Read the model definition and answer for the solid it produces. Units are mm, in the model's axes. A direction names the side the tool comes from. Coordinates: 2 decimals unless noted, no trailing zeros. Order: outer loops, then holes, each group sorted by start corner. A loop starts at its lowest first (then second) coordinate and runs counter-clockwise, first axis right, second up. Notation, with made-up numbers: M 53.5,56.5 L 57.5,56.5 A15 ccw 57.5,80.5 Z; hole C 11,89 d1. An arc over 180 degrees is marked long. Put each result on its own line as item: value.
Autodesk Inventor part; units mm, degrees
ref_plane "YZ Plane" through (0, 0, 0) normal (1, 0, 0) x (0, 1, 0)
ref_plane "XZ Plane" through (0, 0, 0) normal (0, 1, 0) x (-1, 0, 0)
ref_plane "XY Plane" through (0, 0, 0) normal (0, 0, 1) x (1, 0, 0)
sketch "Sketch1" plane through (0, 0, 0) normal (1, 0, 0) x (0, 1, 0)
  line L0 (0, 0) -> (0, -75)
  line L1 (0, -75) -> (3.365, -69.5807)
  line L2 (8.696, -38.0184) -> (0, 0)
  arc A0 (0, -75) -> (5.1288, -67.1329) centre (-33.3696, -47.6401) ccw
  arc A1 (0, -75) -> (8.2317, -57.2892) centre (-44.922, -43.3526) ccw
  arc A2 (8.2317, -57.2892) -> (8.696, -38.0184) centre (-47.0413, -46.3165) ccw
  point P0 (13.3125, -58.2014)
  dimension "d0" = 75
extrude "Extrusion1" add sketch "Sketch1" along normal blind 300 contours L2 A2 A1 L1 L0
sketch "Sketch2" plane through (0, 0, 0) normal (-1, 0, 0) x (0, 0, 1)
  line L0 (-99.8775, 0) -> (-66.8775, 0)
  line L1 (0, 0) -> (-75, 0)
  line L2 (-30.8596, 6.469) -> (-38.8596, 6.469)
  line L3 (-38.8596, 6.469) -> (-38.8596, 0.469)
  line L4 (-38.8596, 0.469) -> (-30.8596, 0.469)
  line L5 (-30.8596, 0.469) -> (-30.8596, 6.469)
  arc A0 (-87.3159, 9.7453) -> (-75, 0) centre (-67.8231, -28.7531) ccw
  line L6 (-75, 0) -> (-36, 0)
  dimension "d3" = 33
  dimension "d4" = 8
  dimension "d5" = 6
  dimension "d15" = 39
extrude "Extrusion2" add sketch "Sketch2" along normal blind 30
sketch "Sketch3" plane through (0, 6.469, -56.2845) normal (0, 1, 0) x (1, 0, 0)
  line L0 (-30, -17.4249) -> (-30, -25.4249)
  circle A0 centre (-30, -21.4249) radius 24
  circle A1 centre (-30, -21.4249) radius 5.25
  point P0 (0, -56.2845)
  dimension "d8" = 48
  dimension "d9" = 10.5
extrude "Extrusion3" add sketch "Sketch3" against normal blind 10
sketch "Sketch4" plane through (0, 6.469, -56.2845) normal (0, 1, 0) x (1, 0, 0)
  line L0 (-30, -17.4249) -> (-30, -25.4249)
  circle A0 centre (-30, -21.4249) radius 5.25
  point P0 (0, -56.2845)
  dimension "d12" = 10.5
extrude "Extrusion4" cut sketch "Sketch4" against normal blind 30
properties part number "elevator"
Q1. Find section A-A on x = -30. Write down the section's boundary in (y, z), plus the area to 3 significant figures.
Answers below:
outline: M -3.53,-58.86 L 6.47,-58.86 L 6.47,-40.11 L -3.53,-40.11 Z; M -3.53,-29.61 L 6.47,-29.61 L 6.47,-10.86 L -3.53,-10.86 Z
area: 375 mm^2
Q2. Given pin 1 (3 mm diameter, centred on y = 3.5, z = -19, fed in from -X); pin 2 (6 mm diameter, centred on y = 0, z = -33.5, fed in from -X); pin 3 (8 mm diameter, centred on x = 128, z = -26, fed in from +Y); pin 4 (10 mm diameter, centred on x = 243.5, z = -35.5, fed in from -Y), each flat-ended and moving along its own axis, determine where each tip first touches the part or whether it passes through.
Answers below:
pin 1: stops at x = -49.23
pin 2: stops at x = -54
pin 3: stops at y = 6.86
pin 4: stops at y = 0
Q3. A tool of negligible diameter and unlimited length cuts with its end or side. For faces 1 (the face through (-3, 3, -30.86)), 2 (the face through (-27, 6.469, -40)), 3 (the face through (148, 0, -37)), from which of +Z, -Z, +X, -X, +Y, -Y can it reach the whole face along a straight path? Write none if from no direction.
Answers below:
face 1: +Z, +Y, -Y
face 2: +Z, -Z, -X, +Y
face 3: +Z, -Z, +X, -Y
Q4. Find section B-B on x = 118.5. Write down the section's boundary in (y, z) (1 decimal).
Answers below:
outline: M 0,-75 L 3.4,-69.6 A55 ccw 8.2,-57.3 A56.4 ccw 8.7,-38 L 0,0 Z
Q5. Find section C-C on z = -62. Write down the section's boundary in (x, y).
Answers below:
outline: M 0,0 L 300,0 L 300,6.77 L 0,6.77 Z
Q6. For a pull along X with two mould halves and no side action, classify faces 4 (the face through (-3, 0.469, -35)), 5 (the face through (147.9, 9.297, -47.538)), 6 (the face through (300, 4, -45)), 7 (the face through (-34.17, 1.54, -31.67)) as +X half, -X half, draft (parallel to the pull), parting line (faces both ways), or undercut.
Answers below:
face 4: undercut
face 5: draft
face 6: +X half
face 7: undercut
Q7. Consider line 1 along Z through (x, y) = (-30, 4.25); line 2 along X through (y, z) = (1.5, -34); line 3 along X through (y, z) = (6.5, -58). Determine where each line is inside the solid, lowest interval first.
Answers below:
line 1: z = -58.86 to -40.11, -29.61 to -10.86
line 2: x = -53.98 to -35.18, -24.82 to 300
line 3: x = 0 to 300
